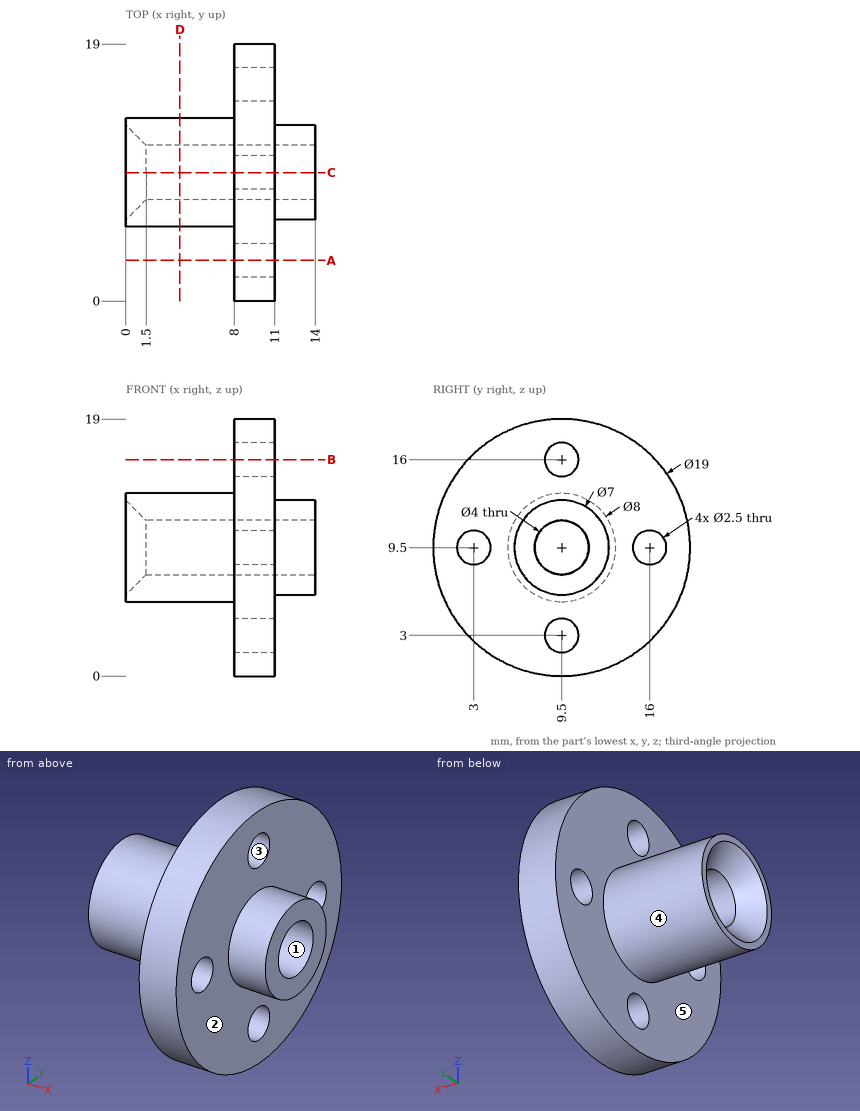
Here's the drawing with two shaded views (mm, measured from the low corner). I have some questions. A direction names the side the tool comes from. Round coordinates to 2 decimals unless told otherwise and drop trailing zeros. Order: outer loops, then holes, each group sorted by start corner. A loop starts at its lowest first (then second) coordinate and runs counter-clockwise, first axis right, second up. Notation, with made-up numbers: (74, 82.5) -> (132, 82.5) arc R33 cw to (132, 120.5) -> close; hole circle Ø3 at (29, -21.75). An arc over 180 degrees is marked (long way). Use a Markdown table: item, result. Add a question column.
(1) Suppose I cut it at D-D, the plane x = 4. Please give me the cut outline in (y, z), and give its area (3 significant figures).
(2) For the marked faces 1 and 2, which set-ups out of +Z, -Z, +X, -X, +Y, -Y let a thin tool reach every point of the face, with its end or its side?
(3) If we mould it in two halves opening along Z, with no side actions, what happens to the marked faces 3, 4 and 5? For each: released by +Z, released by -Z, zero draft, split by the parting line, or undercut.
(4) Suppose I cut it at A-A, the plane y = 3. Please give me the cut outline in (x, z).
(5) I need wall thicknesses on line 1 along Y through (x, z) = (10, 9.5); line 2 along X through (y, z) = (9.25, 1.5); line 3 along Y through (x, z) = (1.25, 11). Which ranges of each line are inside material? Lowest first, please.
(6) For pin 1 Ø3 at (y, z) = (3, 9.5) entering from -X; pin 2 Ø1 at (x, z) = (10, 4) entering from -Y; pin 3 Ø3 at (y, z) = (9.5, 3) entering from +X, each with a flat end and sliding along its axis, tell me the tip position at first contact or that it passes through.
(7) Suppose I cut it at C-C, the plane y = 9.5. Please give me the cut outline in (x, z), and give its area (4 significant figures).
Verdict:
| question | item | result |
|---|---|---|
| 1 | outline | circle Ø8 at (9.5, 9.5); hole circle Ø4 at (9.5, 9.5) |
| 1 | area | 37.7 mm2 |
| 2 | face 1 | +X, -X |
| 2 | face 2 | +X |
| 3 | face 3 | undercut |
| 3 | face 4 | split by the parting line |
| 3 | face 5 | zero draft |
| 4 | outline | (8, 2.57) -> (11, 2.57) -> (11, 8.25) -> (8, 8.25) -> close; (8, 10.75) -> (11, 10.75) -> (11, 16.43) -> (8, 16.43) -> close |
| 5 | line 1 | 0 to 1.75, 4.25 to 7.5, 11.5 to 14.75, 17.25 to 19 |
| 5 | line 2 | 8 to 11 |
| 5 | line 3 | 5.79 to 7.82, 11.18 to 13.21 |
| 6 | pin 1 | x = 8 |
| 6 | pin 2 | y = 1.42 |
| 6 | pin 3 | x = 11 |
| 7 | outline | (0, 5.5) -> (8, 5.5) -> (8, 4.25) -> (11, 4.25) -> (11, 6) -> (14, 6) -> (14, 7.5) -> (1.5, 7.5) -> (0, 6) -> close; (0, 13) -> (1.5, 11.5) -> (14, 11.5) -> (14, 13) -> (11, 13) -> (11, 14.75) -> (8, 14.75) -> (8, 13.5) -> (0, 13.5) -> close; (8, 0) -> (11, 0) -> (11, 1.75) -> (8, 1.75) -> close; (8, 17.25) -> (11, 17.25) -> (11, 19) -> (8, 19) -> close |
| 7 | area | 68.75 mm2 |
